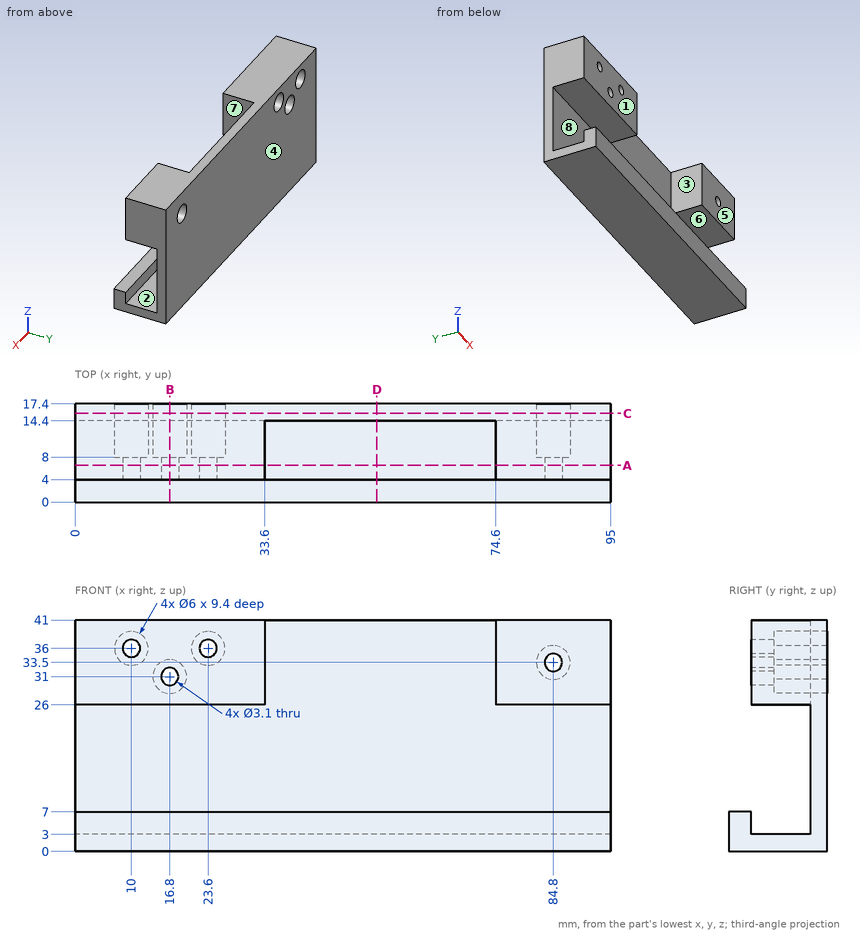
The drawing under review shows one solid part. Ordinate dimensions are in mm from its lowest x, y, z. A direction names the side the tool comes from. Coordinates: 2 decimals unless noted, no trailing zeros. Order: outer loops, then holes, each group sorted by start corner. A loop starts at its lowest first (then second) coordinate and runs counter-clockwise, first axis right, second up. Notation, with made-up numbers: (59.5, 56) -> (76.5, 56) arc R28 cw to (76.5, 85) -> close; hole circle Ø8 at (83, -38). An arc over 180 degrees is marked (long way). Answer in a Markdown table with one row per item.
(1) Consider section A-A (y = 6.5). Write out the cut boundary in (x, z).
Answers:
| item | result |
|---|---|
| outline | (0, 0) -> (95, 0) -> (95, 3) -> (0, 3) -> close; (0, 26) -> (33.6, 26) -> (33.6, 41) -> (0, 41) -> close; (74.6, 26) -> (95, 26) -> (95, 41) -> (74.6, 41) -> close; hole circle Ø3.1 at (10, 36); hole circle Ø3.1 at (16.8, 31); hole circle Ø3.1 at (23.6, 36); hole circle Ø3.1 at (84.8, 33.5) |
(2) Consider section D-D (x = 53.5). Write out the cut boundary in (y, z).
Answers:
| item | result |
|---|---|
| outline | (0, 0) -> (17.4, 0) -> (17.4, 41) -> (14.4, 41) -> (14.4, 3) -> (4, 3) -> (4, 7) -> (0, 7) -> close |
(3) Consider section B-B (x = 16.8). Write out the cut boundary in (y, z).
Answers:
| item | result |
|---|---|
| outline | (0, 0) -> (17.4, 0) -> (17.4, 28) -> (8, 28) -> (8, 29.45) -> (4, 29.45) -> (4, 26) -> (14.4, 26) -> (14.4, 3) -> (4, 3) -> (4, 7) -> (0, 7) -> close; (4, 32.55) -> (8, 32.55) -> (8, 34) -> (17.4, 34) -> (17.4, 41) -> (4, 41) -> close |
(4) Insertion check: pin 1 (1.8 mm diameter, centred on x = 25, z = 37, fed in from +Y); pin 2 (4 mm diameter, centred on x = 15, z = 22.5, fed in from -Y); pin 3 (5 mm diameter, centred on x = 23.6, z = 36, fed in from -Y). Each pin has a flat end and moves straight along its axis. Give the tip position at first contact, or say it passes through.
Answers:
| item | result |
|---|---|
| pin 1 | y = 8 |
| pin 2 | y = 14.4 |
| pin 3 | y = 4 |
(5) Consider section C-C (y = 15.75). Write out the cut boundary in (x, z), plus the area to 3 significant figures.
Answers:
| item | result |
|---|---|
| outline | (0, 0) -> (95, 0) -> (95, 41) -> (0, 41) -> close; hole circle Ø6 at (10, 36); hole circle Ø6 at (16.8, 31); hole circle Ø6 at (23.6, 36); hole circle Ø6 at (84.8, 33.5) |
| area | 3,780 mm² |
(6) Wall thickness on line 1 along X through (y, z) = (6.5, 36); line 2 along Z through (x, y) = (23.6, 7.1); line 3 along Z through (x, y) = (84.8, 7.2): over which ranges is each line inside the solid? List them lowest first.
Answers:
| item | result |
|---|---|
| line 1 | 0 to 8.45, 11.55 to 22.05, 25.15 to 33.6, 74.6 to 95 |
| line 2 | 0 to 3, 26 to 34.45, 37.55 to 41 |
| line 3 | 0 to 3, 26 to 31.95, 35.05 to 41 |
(7) The part is to be moulded in two halves that separate along Y. For the marked faces 1, 2, 3 and 4, say which applies: +Y half, -Y half, draft (parallel to the pull), parting line (faces both ways), or undercut.
Answers:
| item | result |
|---|---|
| face 1 | -Y half |
| face 2 | undercut |
| face 3 | draft |
| face 4 | +Y half |
(8) Machinability: for the marked faces 5, 6, 7 and 8, which of the approach directions +Z, -Z, +X, -X, +Y, -Y give a long, thin tool a straight path to every point of the face, cutting with its end or side? Answer none if there is none.
Answers:
| item | result |
|---|---|
| face 5 | +Z, +X, -X, -Y |
| face 6 | +X, -X, -Y |
| face 7 | +Z, -Y |
| face 8 | none |
